Input: part model. Units: mm. Frame: model coordinates. Face numbers are marked on the shaded views. A direction names the side the tool comes from. Round coordinates to 2 decimals unless told otherwise and drop trailing zeros. Write each loop counter-clockwise with the first axis right and the second up, starting at its lowest first coordinate (ties: lowest second). Pieces come first, ordered by that corner, then holes. Notation, with made-up numbers: (-39, 80.5) -> (-34, 80.5) arc R16 cw to (-34, 89.5) -> close; hole circle Ø5 at (-24.5, -10.75). An arc over 180 degrees is marked (long way). Write item = value, one per line.
```python
from build123d import *

# Parameters (mm, degrees)
F1_DEPTH = 25.4
F2_R     = 6.096
F3_DEPTH = 7.62


with BuildPart() as f1:
    # F0 (on Top) → F1 (new body)
    with BuildSketch(Plane.XY):
        with BuildLine():
            ThreePointArc((0, 8.89), (8.89, 0), (0, -8.89))
            Line((0, -8.89), (0, -13.97))
            ThreePointArc((0, -13.97), (13.97, 0), (0, 13.97))
            Line((0, 13.97), (0, 8.89))
        make_face()
    extrude(amount=F1_DEPTH)

    # F2 (on face) → F3 (join)
    with BuildSketch(Plane(origin=(0, 0, 0), x_dir=(1, 0, 0), z_dir=(0, 0, -1))):
        with BuildLine():
            Line((100.33, 8.89), (10.776307, 8.89))
            ThreePointArc((10.776307, 8.89), (13.97, 0), (10.776307, -8.89))
            Line((10.776307, -8.89), (100.33, -8.89))
            Line((100.33, -8.89), (100.33, 8.89))
        make_face()
        with Locations((31.75, 0)):
            Circle(F2_R, mode=Mode.SUBTRACT)
        with Locations((87.63, 0)):
            Circle(F2_R, mode=Mode.SUBTRACT)
    extrude(amount=-F3_DEPTH)


solid = f1.part
```
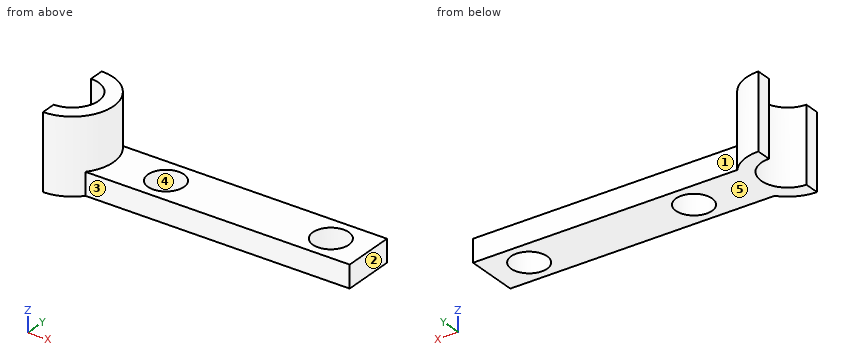
1) Cut plane B-B (x = 87.63). Return the cut outline in (y, z), and give its area (3 significant figures).
Solutions:
outline = (-8.89, 0) -> (-6.1, 0) -> (-6.1, 7.62) -> (-8.89, 7.62) -> close; (6.1, 0) -> (8.89, 0) -> (8.89, 7.62) -> (6.1, 7.62) -> close
area = 42.6 mm^2
2) Cut plane A-A (y = 0). Return the cut outline in (x, z), and give its area (3 significant figures).
Solutions:
outline = (8.89, 0) -> (25.65, 0) -> (25.65, 7.62) -> (13.97, 7.62) -> (13.97, 25.4) -> (8.89, 25.4) -> close; (37.85, 0) -> (81.53, 0) -> (81.53, 7.62) -> (37.85, 7.62) -> close; (93.73, 0) -> (100.33, 0) -> (100.33, 7.62) -> (93.73, 7.62) -> close
area = 601 mm^2
3) First-contact query: P1, Ø8, axis at y = -1.5, z = 14, coming from the +X side; P2, Ø5, axis at y = -10, z = 16.5, coming from the +X side; P3, Ø6, axis at x = 21, z = 9, coming from the +Y side. Flat tips, straight axial feed; report the tip coordinate or a pass-through.
Solutions:
P1 = 13.97
P2 = 11.79
P3 = 8.89
4) Cut plane C-C (z = 6.75). Return the cut outline in (x, y), and give its area (3 significant figures).
Solutions:
outline = (0, -13.97) arc R13.97 ccw to (10.78, -8.89) -> (100.33, -8.89) -> (100.33, 8.89) -> (10.78, 8.89) arc R13.97 ccw to (0, 13.97) -> (0, 8.89) arc R8.89 cw to (0, -8.89) -> close; hole circle Ø12.19 at (31.75, 0); hole circle Ø12.19 at (87.63, 0)
area = 1,500 mm^2
5) Cut plane D-D (z = 19.25). Return the cut outline in (x, y).
Solutions:
outline = (0, -13.97) arc R13.97 ccw to (0, 13.97) -> (0, 8.89) arc R8.89 cw to (0, -8.89) -> close
6) Draft query along Y for the marked faces 3, 4 and 5. Return one class per face: +Y half, -Y half, draft (parallel to the pull), parting line (faces both ways), or undercut.
Solutions:
face_3 = -Y half
face_4 = undercut
face_5 = draft
7) Access query for the marked faces 1 and 2. Directions: +Z, -Z, +X, -X, +Y, -Y. A direction counts if a zero-diameter tool reaches every point of the face in a straight line with its end or side. Return the directions, or none.
Solutions:
face_1 = +Z, -Z, +X, +Y
face_2 = +Z, -Z, +X, +Y, -Y
8) Line query: L1, parallel to X at y = 0, z = 4; L2, parallel to X at y = -0.5, z = 2.5; L3, parallel to Y at x = 31.75, z = 3.25. Output: solid intervals per line, ascending. Write a range as from..to.
Solutions:
L1 = 8.89..25.65, 37.85..81.53, 93.73..100.33
L2 = 8.88..25.67, 37.83..81.55, 93.71..100.33
L3 = -8.89..-6.1, 6.1..8.89
